```python
from build123d import *

# Parameters (mm, degrees)
CROQUIS1_W              = 300
CROQUIS1_H              = 210
SALIENTE_EXTRUIR1_DEPTH = 3
CROQUIS3_R              = 2.5
CORTAR_EXTRUIR1_DEPTH   = 4
CROQUIS4_R              = 4
CORTAR_EXTRUIR2_DEPTH   = 4


with BuildPart() as part:
    # Croquis1 → Saliente-Extruir1 (new body)
    with BuildSketch(Plane.XY):
        Rectangle(CROQUIS1_W, CROQUIS1_H)
    extrude(amount=SALIENTE_EXTRUIR1_DEPTH)

    # Croquis3 → Cortar-Extruir1 (cut, through all)
    with BuildSketch(Plane.XY.offset(3)):
        with Locations((0, 95)):
            Circle(CROQUIS3_R)
        with Locations((-140, 0)):
            Circle(CROQUIS3_R)
        with Locations((100, 95)):
            Circle(CROQUIS3_R)
        with Locations((-100, 95)):
            Circle(CROQUIS3_R)
        with Locations((-140, 80)):
            Circle(CROQUIS3_R)
        with Locations((-140, -80)):
            Circle(CROQUIS3_R)
        with Locations((100, -95)):
            Circle(CROQUIS3_R)
        with Locations((-100, -95)):
            Circle(CROQUIS3_R)
        with Locations((0, -95)):
            Circle(CROQUIS3_R)
        with Locations((140, -80)):
            Circle(CROQUIS3_R)
        with Locations((140, 80)):
            Circle(CROQUIS3_R)
        with Locations((140, 0)):
            Circle(CROQUIS3_R)
    extrude(amount=-CORTAR_EXTRUIR1_DEPTH, mode=Mode.SUBTRACT)

    # Croquis4 → Cortar-Extruir2 (cut, through all)
    with BuildSketch(Plane.XY.offset(3)):
        with Locations((-60, 0)):
            Circle(CROQUIS4_R)
        with Locations((60, 0)):
            Circle(CROQUIS4_R)
    extrude(amount=-CORTAR_EXTRUIR2_DEPTH, mode=Mode.SUBTRACT)


solid = part.part
```
Check sheet for the modelled part. Datum: model origin and axes. Units: mm. Round coordinates to 2 decimals unless told otherwise and drop trailing zeros. Write each loop counter-clockwise with the first axis right and the second up, starting at its lowest first coordinate (ties: lowest second). Pieces come first, ordered by that corner, then holes. Notation, with made-up numbers: M -22,30.25 L -14,30.25 A7 cw -14,39.25 Z; hole C 38.25,45.25 d11. An arc over 180 degrees is marked long. Write item = value, one per line. Start each with the question number.
1. Section check A-A, the plane x = -60. Record the cut outline in (y, z).
2. Release check for a two-part mould opening along X. For faces 1 (the cylindrical face through (63.815, 1.201, 1.521)), 2 (the flat face through (-2, 1, 0)) record: pulls with the +X half, pulls with the -X half, needs draft (parallel to the pull), parting line crosses it, or undercut.
3. Section check B-B, the plane x = 61. Record the cut outline in (y, z), then the cut area to 3 significant figures.
4. Scan lines: line 1 (Y direction, x = -140, z = 1.65); line 2 (X direction, y = -94.5, z = 0.65); line 3 (X direction, y = 3.5, z = 2.3). Record each from-to range of solid material in increasing order. Write a range as [from, to].
Results found:
q1.outline = M -105,0 L -4,0 L -4,3 L -105,3 Z; M 4,0 L 105,0 L 105,3 L 4,3 Z
q2.face_1 = undercut
q2.face_2 = needs draft
q3.outline = M -105,0 L -3.87,0 L -3.87,3 L -105,3 Z; M 3.87,0 L 105,0 L 105,3 L 3.87,3 Z
q3.area = 607 mm^2
q4.line_1 = [-105, -82.5], [-77.5, -2.5], [2.5, 77.5], [82.5, 105]
q4.line_2 = [-150, -102.45], [-97.55, -2.45], [2.45, 97.55], [102.45, 150]
q4.line_3 = [-150, -61.94], [-58.06, 58.06], [61.94, 150]
